Source: CAD feature listing. Evaluate the final solid. Frame: model axes, mm. A direction names the side the tool comes from. Coordinates: 2 decimals unless noted, no trailing zeros. Loops run counter-clockwise (first coordinate to the right, second up) from the corner with the lowest first, then second, coordinate; pieces in that order, holes last. Notation, with made-up numbers: M 82,8 L 122,8 A16 ccw 122,18 Z; hole C 58,-1.5 d4. An arc over 180 degrees is marked long. One line per question, with ' | ' between items. Start each with the question number.
1. Mould query, pull axis X, two halves, no side actions, for faces 3 (the flat face through (31, 1, 0)), 4 (the flat face through (32.5, 1, -8)), 5 (the flat face through (29, 1, -8)). Classes: pulls with the +X half, pulls with the -X half, needs draft (parallel to the pull), parting line crosses it, or undercut.
2. Pin query (flat end, axial travel): P1, Ø8, axis at x = 2, z = -18, coming from the -Y side. Return the tip coordinate at first contact, or that it passes through.
3. Section query A-A, the plane z = -6.75. Output: boundary loops of the cut face in (x, y).
4. Ray query, probe 1 along X at (y, z) = (2.75, -13); probe 2 along Z at (x, y) = (-2, 0.2); probe 3 along Z at (x, y) = (-11, 1.4). Return the intervals inside material, ascending.
5. Access query for faces 1 (the flat face through (0, 1, -15.522)), 2 (the flat face through (-3, 3, -16)). Directions: +Z, -Z, +X, -X, +Y, -Y. A direction counts if a zero-diameter tool reaches every point of the face in a straight line with its end or side. Return the directions, or none.
```python
from build123d import *

# Parameters (mm, degrees)
BOSS_EXTRUDE1_DEPTH = 3
CUT_EXTRUDE1_DEPTH  = 4.0000001
SKETCH3_R           = 1.0922
CUT_EXTRUDE2_DEPTH  = 4.0000001
FILLET1_R           = 5
FILLET2_R           = 0.5
CUT_EXTRUDE3_DEPTH  = 4.0000001
FILLET3_R           = 0.5


with BuildPart() as part:
    # Sketch1 → Boss-Extrude1 (new body)
    with BuildSketch(Plane(origin=(0, 0, 0), x_dir=(1, 0, 0), z_dir=(0, 1, 0))):
        with BuildLine():
            Line((0, 0), (-32.5, 0))
            Line((-32.5, 0), (-32.5, 16))
            add(Edge.make_bspline(
                [(0, 20.5), (-32.5, 20.5), (-32.5, 16)],
                knots=[4.71238898, 4.71238898, 4.71238898, 6.283185307, 6.283185307, 6.283185307], degree=2, weights=[1, 0.707106781, 1]))
            Line((0, 20.5), (0, 16))
            Line((0, 16), (0, 0))
        make_face()
    boss_extrude1 = extrude(amount=BOSS_EXTRUDE1_DEPTH)

    # Mirror1: Boss-Extrude1 across plane
    add(boss_extrude1.mirror(Plane(origin=(0, 3, -16), x_dir=(0, 0, 1), z_dir=(-1, 0, 0))))

    # Sketch2 → Cut-Extrude1 (cut, through all)
    with BuildSketch(Plane(origin=(0, 3, 0), x_dir=(1, 0, 0), z_dir=(0, 1, 0))):
        with BuildLine():
            Line((0, 10.25), (0, 12.5))
            add(Edge.make_bspline(
                [(0, 12.5), (-20.26, 12.5), (-20.26, 10.25)],
                knots=[4.71238898, 4.71238898, 4.71238898, 6.283185307, 6.283185307, 6.283185307], degree=2, weights=[1, 0.707106781, 1]))
            Line((-20.26, 10.25), (-20.26, 0))
            Line((-20.26, 0), (0, 0))
            Line((0, 0), (0, 10.25))
        make_face()
        with BuildLine():
            Line((20.26, 0), (20.26, 10.25))
            add(Edge.make_bspline(
                [(20.26, 10.25), (20.26, 12.5), (0, 12.5)],
                knots=[3.141592654, 3.141592654, 3.141592654, 4.71238898, 4.71238898, 4.71238898], degree=2, weights=[1, 0.707106781, 1]))
            Line((0, 12.5), (0, 10.25))
            Line((0, 10.25), (0, 0))
            Line((0, 0), (20.26, 0))
        make_face()
    extrude(amount=-CUT_EXTRUDE1_DEPTH, mode=Mode.SUBTRACT)

    # Sketch3 → Cut-Extrude2 (cut, through all)
    with BuildSketch(Plane.XZ):
        with Locations((25.46, -4.3615)):
            Circle(SKETCH3_R)
        with Locations((-25.34, -4.3615)):
            Circle(SKETCH3_R)
    extrude(amount=-CUT_EXTRUDE2_DEPTH, mode=Mode.SUBTRACT)

    # Fillet1
    fillet1_edges = [part.edges().sort_by_distance(p)[0] for p in [
        (20.26, 1.5, 0),
        (-20.26, 1.5, 0),
    ]]
    fillet(fillet1_edges, radius=FILLET1_R)

    # Fillet2
    fillet2_edges = [part.edges().sort_by_distance(p)[0] for p in [
        (32.5, 1.5, 0),
        (-32.5, 1.5, 0),
    ]]
    fillet(fillet2_edges, radius=FILLET2_R)

    # Sketch4 → Cut-Extrude3 (cut, through all)
    with BuildSketch(Plane.XZ):
        Polygon((29, -1.8215), (29, 0), (-29, 0), (-29, -1.8215), (-29, -15.5215), (29, -15.5215), align=None)
    extrude(amount=-CUT_EXTRUDE3_DEPTH, mode=Mode.SUBTRACT)

    # Fillet3
    fillet3_edges = [part.edges().sort_by_distance(p)[0] for p in [
        (-29, 1.5, 0),
        (29, 1.5, 0),
    ]]
    fillet(fillet3_edges, radius=FILLET3_R)


solid = part.part
```
Taken from the geometry:
1) face 3: needs draft | face 4: pulls with the +X half | face 5: undercut
2) P1: y = 0
3) outline: M -32.5,0 L -29,0 L -29,3 L -32.5,3 Z; M 29,0 L 32.5,0 L 32.5,3 L 29,3 Z
4) probe 1: -32.5 to -29, 29 to 32.5 | probe 2: -20.49 to -15.52 | probe 3: -20.23 to -15.52
5) face 1: +Z, +Y, -Y | face 2: +Z, -Z, +X, -X, +Y
